Could you check a few things on this model? Use its own coordinates, in mm. Give positions to 0.01 mm unless a question says otherwise; leave off trailing zeros. Loops run counter-clockwise (first coordinate to the right, second up) from the corner with the lowest first, then second, coordinate; pieces in that order, holes last. Notation, with made-up numbers: M 43.5,29.5 L 96.5,29.5 A24 cw 96.5,67.5 Z; hole C 11.5,-3.5 d10. An arc over 180 degrees is marked long. Return JSON: item names as keys, results as strings. Group by question number.
1. If we section it at B-B (y = 0): Write out the boundary of the cut face in (x, z), plus the area to 3 significant figures.
2. If we section it at C-C (y = 5): Write out the boundary of the cut face in (x, z), plus the area to 3 significant figures.
3. If we section it at D-D (y = 3.5): Write out the boundary of the cut face in (x, z).
4. If we mould it in two halves opening along X, with no side actions, what happens to faces 1 (the cylindrical face through (-53.75, 0.14, 1.97)), 2 (the flat face through (-37, 0, 4)), 3 (the flat face through (-20, 0, 2)), 4 (the cylindrical face through (-49.498, 0.088, 1.479))? For each: +X half, -X half, draft (parallel to the pull), parting line (faces both ways), or undercut.
5. For pin 1 (1 mm diameter, centred on y = 2, z = 2.5, fed in from -X), with a flat end and sliding along its axis, tell me the tip position at first contact or that it passes through.
6. Please list where these lines run through material, in increasing order: line 1 (Y direction, x = -47.5, z = 1.35); line 2 (X direction, y = -1.25, z = 1.5); line 3 (Y direction, x = -47, z = 3.6).
7. If we section it at A-A (z = 0.35): Write out the boundary of the cut face in (x, y).
```python
from build123d import *

# Parameters (mm, degrees)
CYLINDER004_R     = 2
CYLINDER004_DEPTH = 4
BOX006_W          = 27.5
BOX006_H          = 12.5
BOX006_DEPTH      = 4
TUBE001_R         = 6.25
TUBE001_DEPTH     = 4
CHAMFER_SIZE      = 1


with BuildPart() as obj1:
    # Cylinder004 → Cylinder004 (new body)
    with BuildSketch(Plane(origin=(-47.5, 0, 0), x_dir=(1, 0, 0), z_dir=(0, 0, 1))):
        Circle(CYLINDER004_R)
    extrude(amount=CYLINDER004_DEPTH)


with BuildPart() as arm001:
    # Box006 → Box006 (new body)
    with BuildSketch(Plane(origin=(-47.5, -6.25, 0), x_dir=(1, 0, 0), z_dir=(0, 0, 1))):
        with Locations((13.75, 6.25)):
            Rectangle(BOX006_W, BOX006_H)
    extrude(amount=BOX006_DEPTH)


with BuildPart() as chamfer_body:
    # Tube001 → Tube001 (new body)
    with BuildSketch(Plane(origin=(-47.5, 0, 0), x_dir=(1, 0, 0), z_dir=(0, 0, 1))):
        Circle(TUBE001_R)
    extrude(amount=TUBE001_DEPTH)

    # Fusion001: union Arm001
    add(arm001.part)

    # Cut001: cut obj1
    add(obj1.part, mode=Mode.SUBTRACT)

    # Chamfer
    chamfer_edges = [chamfer_body.edges().sort_by_distance(p)[0] for p in [
        (-46.085786, 1.414214, 4),
        (-49.5, 0, 4),
        (-46.085786, -1.414214, 4),
    ]]
    chamfer(chamfer_edges, length=CHAMFER_SIZE)


solid = chamfer_body.part
```
Answer:
{
 "1": {"outline": "M -53.75,0 L -49.5,0 L -49.5,3 L -50.5,4 L -53.75,4 Z; M -45.5,0 L -20,0 L -20,4 L -44.5,4 L -45.5,3 Z", "area": "118 mm²"},
 "2": {"outline": "M -51.25,0 L -20,0 L -20,4 L -51.25,4 Z", "area": "125 mm²"},
 "3": {"outline": "M -52.68,0 L -20,0 L -20,4 L -52.68,4 Z"},
 "4": {"face 1": "-X half", "face 2": "draft", "face 3": "+X half", "face 4": "undercut"},
 "5": {"pin 1": "stops at x = -53.57"},
 "6": {"line 1": "y = -6.25 to -2, 2 to 6.25", "line 2": "x = -53.62 to -49.06, -45.94 to -20", "line 3": "y = -6.25 to -2.55, 2.55 to 6.25"},
 "7": {"outline": "M -47.5,-6.25 L -20,-6.25 L -20,6.25 L -47.5,6.25 A6.25 ccw Z; hole C -47.5,0 d4"}
}
